Verification items for this drawing (mm, ordinates from the low corner). A direction names the side the tool comes from. Round coordinates to 2 decimals unless told otherwise and drop trailing zeros. Order: outer loops, then holes, each group sorted by start corner. A loop starts at its lowest first (then second) coordinate and runs counter-clockwise, first axis right, second up. Notation, with made-up numbers: (-26, -4.5) -> (-22, -4.5) arc R16 cw to (-22, 21.5) -> close; hole circle Ø1 at (78, -32.75). An arc over 180 degrees is marked (long way). Put each result on its own line as item: value.
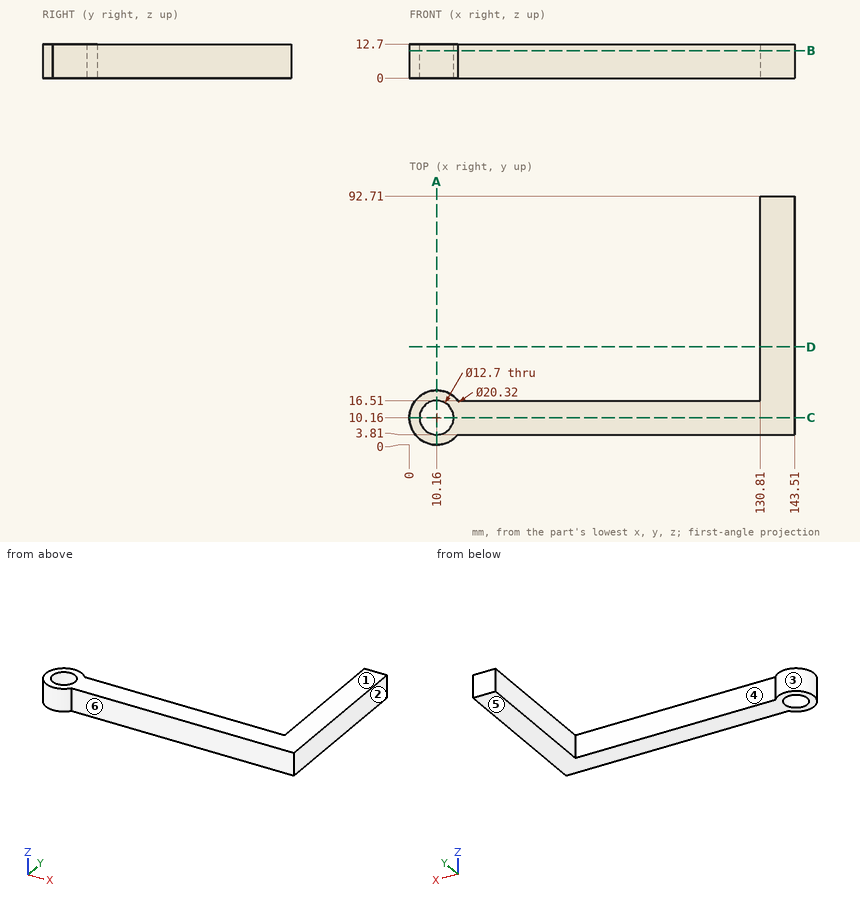
Item 1: Section check A-A on x = 10.16. Record the boundary of the cut face in (y, z), then the cut area to 3 significant figures.
Check sheet entries:
outline: (0, 0) -> (3.81, 0) -> (3.81, 12.7) -> (0, 12.7) -> close; (16.51, 0) -> (20.32, 0) -> (20.32, 12.7) -> (16.51, 12.7) -> close
area: 96.8 mm^2
Item 2: Release check for a two-part mould opening along X. For the marked faces 1, 2 and 3 record: +X half, -X half, draft (parallel to the pull), parting line (faces both ways), or undercut.
Check sheet entries:
face 1: draft
face 2: +X half
face 3: undercut
Item 3: Material ranges on L1, parallel to Y at x = 10.16, z = 7; L2, parallel to X at y = 30, z = 0.75; L3, parallel to X at y = 17.5, z = 2.5, recorded low to high. Write a range as [from, to].
Check sheet entries:
L1: y = [0, 3.81], [16.51, 20.32]
L2: x = [130.81, 143.51]
L3: x = [3.14, 17.18], [130.81, 143.51]
Item 4: Section check D-D on y = 36.5. Record the boundary of the cut face in (x, z), then the cut area to 3 significant figures.
Check sheet entries:
outline: (130.81, 0) -> (143.51, 0) -> (143.51, 12.7) -> (130.81, 12.7) -> close
area: 161 mm^2
Item 5: Section check C-C on y = 10.16. Record the boundary of the cut face in (x, z).
Check sheet entries:
outline: (0, 0) -> (3.81, 0) -> (3.81, 12.7) -> (0, 12.7) -> close; (16.51, 0) -> (143.51, 0) -> (143.51, 12.7) -> (16.51, 12.7) -> close
Item 6: Tool access check on the marked faces 4, 5 and 6. Record the directions out of +Z, -Z, +X, -X, +Y, -Y that give a thin tool (end or side, any length) a straight path to the whole face; none if there is none.
Check sheet entries:
face 4: +Z, -Z, +Y
face 5: -Z, +X, -X, +Y, -Y
face 6: +Z, -Z, +X, -Y
Item 7: Section check B-B on z = 10.25. Record the boundary of the cut face in (x, y).
Check sheet entries:
outline: (18.09, 3.81) -> (143.51, 3.81) -> (143.51, 92.71) -> (130.81, 92.71) -> (130.81, 16.51) -> (18.09, 16.51) arc R10.16 ccw (long way) to start; hole circle Ø12.7 at (10.16, 10.16)
Item 8: Gauge pin test, flat ends, axial feed: pin 1 Ø6.5 at (x, z) = (95, 7) entering from +Y; pin 2 Ø4 at (y, z) = (72.5, 4.5) entering from -X. Record the tip position at first contact, or that the pin passes through.
Check sheet entries:
pin 1: stops at y = 16.51
pin 2: stops at x = 130.81
